Source: CAD feature listing. Evaluate the final solid. Frame: model axes, mm. Round coordinates to 2 decimals unless told otherwise and drop trailing zeros. Write each loop counter-clockwise with the first axis right and the second up, starting at its lowest first coordinate (ties: lowest second). Pieces come first, ordered by that corner, then holes. Notation, with made-up numbers: M -11.5,12 L 4.5,12 A13 ccw 4.5,22 Z; hole C 18.5,51.25 d9. An arc over 180 degrees is marked long. Answer in a Markdown table with one row per item. Add a question column.
Item 1: Cut plane B-B on z = 0. Return loops of the section in (x, y), and give its area (3 significant figures).
Item 2: Cut plane C-C on x = 0. Return loops of the section in (y, z), and give its area (3 significant figures).
Item 3: Contact query for flat-ended pins moving along their axis: pin 1 (0.9 mm diameter, centred on x = -36, y = 2, fed in from +Z); pin 2 (1 mm diameter, centred on y = 2.5, z = 7, fed in from +X); pin 3 (1.4 mm diameter, centred on y = 1, z = -0.5, fed in from -X). Output: stop coordinate, or through.
Item 4: Cut plane D-D on z = -34. Return loops of the section in (x, y).
Item 5: Material intervals for probe 1 along X at (y, z) = (1.85, 1); probe 2 along Z at (x, y) = (41.5, 0.8) (3 decimals); probe 3 along Z at (x, y) = (-20.5, 1.8), sorted ascending.
Item 6: Cut plane A-A on y = 2.1. Return loops of the section in (x, z) (3 decimals).
from build123d import *

# Parameters (mm, degrees)
SKETCH1_R           = 55
BOSS_EXTRUDE1_DEPTH = 3
SKETCH2_R           = 30
CUT_EXTRUDE1_DEPTH  = 3
SKETCH3_W           = 25
SKETCH3_H           = 2.87
CUT_EXTRUDE2_DEPTH  = 3
CIRPATTERN1_COUNT   = 6


with BuildPart() as part:
    # Sketch1 → Boss-Extrude1 (new body)
    with BuildSketch(Plane(origin=(0, 0, 0), x_dir=(1, 0, 0), z_dir=(0, 1, 0))):
        with Locations(Location((0, 0, 0), (0, 0, 270))):
            Circle(SKETCH1_R)
    extrude(amount=BOSS_EXTRUDE1_DEPTH)

    # Sketch2 → Cut-Extrude1 (cut)
    with BuildSketch(Plane(origin=(0, 3, 0), x_dir=(1, 0, 0), z_dir=(0, 1, 0))):
        with Locations(Location((0, 0, 0), (0, 0, 270))):
            Circle(SKETCH2_R)
    extrude(amount=-CUT_EXTRUDE1_DEPTH, mode=Mode.SUBTRACT)

    # Sketch3 → Cut-Extrude2 (cut)
    with BuildSketch(Plane(origin=(0, 3, 0), x_dir=(1, 0, 0), z_dir=(0, 1, 0))):
        with Locations((-30, 0)):
            Rectangle(SKETCH3_W, SKETCH3_H)
    cut_extrude2 = extrude(amount=-CUT_EXTRUDE2_DEPTH, mode=Mode.SUBTRACT)

    # CirPattern1: Cut-Extrude2 ×6 about axis
    cirpattern1_axis = Axis((0, 0, 0), (0, 1, 0))
    for i in range(1, CIRPATTERN1_COUNT):
        add(cut_extrude2.rotate(cirpattern1_axis, i * 360 / CIRPATTERN1_COUNT), mode=Mode.SUBTRACT)


solid = part.part
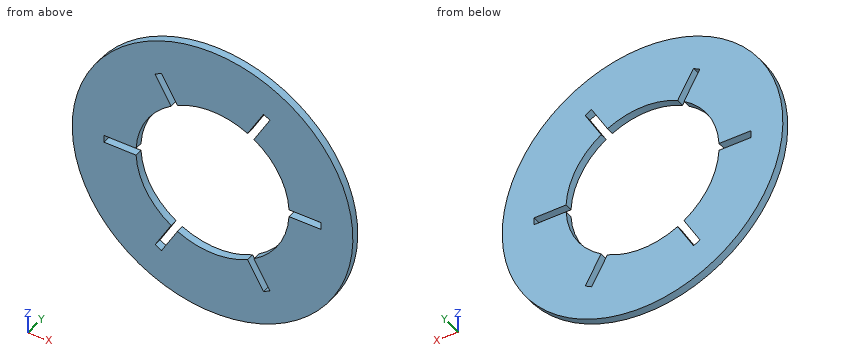
Results below:
| question | item | result |
|---|---|---|
| 1 | outline | M -55,0 L -42.5,0 L -42.5,3 L -55,3 Z; M 42.5,0 L 55,0 L 55,3 L 42.5,3 Z |
| 1 | area | 75.0 mm2 |
| 2 | outline | M 0,-55 L 3,-55 L 3,-30 L 0,-30 Z; M 0,30 L 3,30 L 3,55 L 0,55 Z |
| 2 | area | 150 mm2 |
| 3 | pin 1 | z = 41.97 |
| 3 | pin 2 | x = 54.61 |
| 3 | pin 3 | x = -55 |
| 4 | outline | M -43.23,0 L -21.29,0 L -21.29,3 L -43.23,3 Z; M -17.97,0 L 17.97,0 L 17.97,3 L -17.97,3 Z; M 21.29,0 L 43.23,0 L 43.23,3 L 21.29,3 Z |
| 5 | probe 1 | -54.99 to -42.5, 42.5 to 54.99 |
| 5 | probe 2 | -36.094 to -1.435, 1.435 to 36.094 |
| 5 | probe 3 | -51.04 to -37.24, -32.64 to -21.9, 21.9 to 32.64, 37.24 to 51.04 |
| 6 | outline | C 0,0 d110; hole M -42.5,-1.435 L -29.966,-1.435 A30 ccw -16.226,-25.234 L -22.493,-36.089 L -20.007,-37.524 L -13.74,-26.669 A30 ccw 13.74,-26.669 L 20.007,-37.524 L 22.493,-36.089 L 16.226,-25.234 A30 ccw 29.966,-1.435 L 42.5,-1.435 L 42.5,1.435 L 29.966,1.435 A30 ccw 16.226,25.234 L 22.493,36.089 L 20.007,37.524 L 13.74,26.669 A30 ccw -13.74,26.669 L -20.007,37.524 L -22.493,36.089 L -16.226,25.234 A30 ccw -29.966,1.435 L -42.5,1.435 Z |
